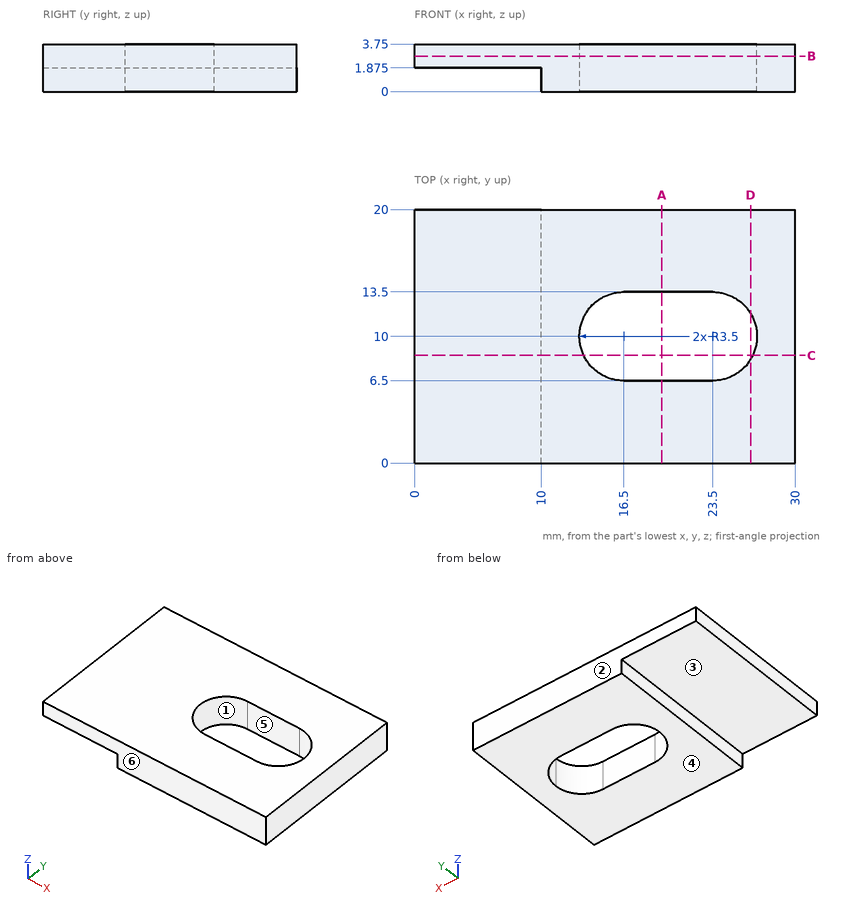
Print and shaded views of the part. All mm, measured from the part's lowest x, y and z. A direction names the side the tool comes from. Round coordinates to 2 decimals unless told otherwise and drop trailing zeros. Order: outer loops, then holes, each group sorted by start corner. A loop starts at its lowest first (then second) coordinate and runs counter-clockwise, first axis right, second up.
Q1. Drop flat-ended pins along their axis: pin 1 (6 mm diameter, centred on x = 11.5, y = 13, fed in from -Z); pin 2 (8 mm diameter, centred on x = 4, y = 11.5, fed in from -Z) (3 decimals). Give the stop position or say it passes through.
Q2. Slice it at A-A (x = 19.5). Write the cut outline in (y, z).
Q3. Two-plate mould, pull along Y, no slides. Class the marked faces 4, 5 and 6: pulls with the +Y half, pulls with the -Y half, needs draft (parallel to the pull), parting line crosses it, or undercut.
Q4. Slice it at C-C (y = 8.5). Write the cut outline in (x, z) (3 decimals).
Q5. Slice it at B-B (z = 2.8). Write the cut outline in (x, y).
Q6. Which spindle directions (+Z, -Z, +X, -X, +Y, -Y) get a long thin tool onto all of the face, cutting with end or side? Do the marked faces 1, 2 and 3. Say none if no direction does.
Q7. Wall check: L1, parallel to Y at x = 17, z = 0.4; L2, parallel to X at y = 12.25, z = 1.6; L3, parallel to Z at x = 5.75, y = 12.25 (3 decimals). Give the ranges that are in metal, low to high.
Q8. Slice it at D-D (x = 26.5). Write the cut outline in (y, z), and give its area (3 significant figures).
Results below:
1. pin 1: stops at z = 0
1. pin 2: stops at z = 1.875
2. outline: (0, 0) - (6.5, 0) - (6.5, 3.75) - (0, 3.75) - close; (13.5, 0) - (20, 0) - (20, 3.75) - (13.5, 3.75) - close
3. face 4: needs draft
3. face 5: undercut
3. face 6: pulls with the -Y half
4. outline: (0, 1.875) - (10, 1.875) - (10, 0) - (13.338, 0) - (13.338, 3.75) - (0, 3.75) - close; (26.662, 0) - (30, 0) - (30, 3.75) - (26.662, 3.75) - close
5. outline: (0, 0) - (30, 0) - (30, 20) - (0, 20) - close; hole (16.5, 6.5) - (23.5, 6.5) arc R3.5 ccw to (27, 10) arc R3.5 ccw to (23.5, 13.5) - (16.5, 13.5) arc R3.5 ccw to start
6. face 1: +Z, -Z
6. face 2: +Z, -Z, +X, -X, +Y
6. face 3: -Z, -X, +Y, -Y
7. L1: y = 0 to 6.5, 13.5 to 20
7. L2: x = 10 to 13.82, 26.18 to 30
7. L3: z = 1.875 to 3.75
8. outline: (0, 0) - (8.2, 0) - (8.2, 3.75) - (0, 3.75) - close; (11.8, 0) - (20, 0) - (20, 3.75) - (11.8, 3.75) - close
8. area: 61.5 mm2
